from build123d import *

# Parameters (mm, degrees)
SKETCH1_W              = 25.4
SKETCH1_H              = 50.8
BASE_FLANGE1_DEPTH     = 25.4
SKETCHED_BEND2_DEPTH   = 25.4
SKETCHED_BEND2_2_DEPTH = 25.4


# Read off the part's stored shape, not the designer's step: Sketched Bend2
# Sheet-metal steps are written as plain solids
with BuildPart() as part:
    # Sketch1 → Base-Flange1 (new body)
    with BuildSketch(Plane.XY):
        with Locations((12.7, 25.4)):
            Rectangle(SKETCH1_W, SKETCH1_H)
    extrude(amount=-BASE_FLANGE1_DEPTH)

    # Sketched Bend2 outline → Sketched Bend2 (cut)
    with BuildSketch(Plane.YZ):
        with BuildLine():
            Line((50.8, -25.4), (50.8, -24.950657177))
            ThreePointArc((50.8, -24.950657177), (48.094844213, -25.287472556), (45.37112433, -25.4))
            Line((45.37112433, -25.4), (50.8, -25.4))
        make_face()
        Polygon((50.8, 0), (48.626141092, 0), (50.8, -12.328566501), align=None)
    extrude(amount=SKETCHED_BEND2_DEPTH, mode=Mode.SUBTRACT)

    # Sketched Bend2 2 outline → Sketched Bend2 2 (add)
    with BuildSketch(Plane.YZ):
        with BuildLine():
            Line((52.958756408, -24.57148247), (50.8, -12.328566501))
            Line((50.8, -12.328566501), (50.8, -24.950657177))
            ThreePointArc((50.8, -24.950657177), (50.95255485, -24.924861858), (51.104987157, -24.898352004))
            Line((51.104987157, -24.898352004), (52.958756408, -24.57148247))
        make_face()
        with BuildLine():
            Line((48.548092695, 0.442634457), (46.694323444, 0.115764922))
            ThreePointArc((46.694323444, 0.115764922), (46.03525109, 0.028996401), (45.37112433, 0))
            Line((45.37112433, 0), (48.626141092, 0))
            Line((48.626141092, 0), (48.548092695, 0.442634457))
        make_face()
    extrude(amount=SKETCHED_BEND2_2_DEPTH)


solid = part.part
The model under review builds one solid part; all positions refer to its coordinate system, in mm. A direction names the side the tool comes from. Give positions to 0.01 mm unless a question says otherwise; leave off trailing zeros. Write each loop counter-clockwise with the first axis right and the second up, starting at its lowest first coordinate (ties: lowest second). Pieces come first, ordered by that corner, then holes.
1. Wall thickness on L1, parallel to Z at x = 6.5, y = 28; L2, parallel to Y at x = 7.25, z = -9.5; L3, parallel to Y at x = 9, z = -18.5: over which ranges is each line inside the solid? List them lowest first.
2. Add section B-B, the plane y = 35. Write out the cut boundary in (x, z).
3. For P1, Ø12, axis at x = 15.5, z = -2.5, coming from the -Y side; P2, Ø4, axis at x = 21, z = -3.5, coming from the +Y side; P3, Ø7.5, axis at x = 7, y = 27, coming from the +Z side, all flat-tipped, find the tip position at first contact; note any pin that passes through.
4. Add section C-C, the plane z = -20. Write out the cut boundary in (x, y).
5. Tool access review of faces 1 (the flat face through (13, 23, 0)), 2 (the flat face through (13, 23, -25.4)): name each direction out of +Z, -Z, +X, -X, +Y, -Y from which nothing blocks a thin tool from reaching the whole face with its end or side.
6. Add section A-A, the plane x = 8.25. Write out the cut boundary in (y, z).
Worked answers:
1. L1: z = -25.4 to 0
1. L2: y = 0 to 50.3
1. L3: y = 0 to 51.89
2. outline: (0, -25.4) - (25.4, -25.4) - (25.4, 0) - (0, 0) - close
3. P1: stops at y = 0
3. P2: stops at y = 49.6
3. P3: stops at z = 0
4. outline: (0, 0) - (25.4, 0) - (25.4, 52.15) - (0, 52.15) - close
5. face 1: +Z, +X, -X, -Y
5. face 2: -Z, +X, -X, +Y, -Y
6. outline: (0, -25.4) - (45.37, -25.4) arc R33.02 ccw to (50.8, -24.95) arc R33.02 ccw to (51.1, -24.9) - (52.96, -24.57) - (48.55, 0.44) - (46.69, 0.12) arc R7.62 cw to (45.37, 0) - (0, 0) - close
